Here's how the part is built. I have some questions about the finished solid (model axes, mm). A direction names the side the tool comes from. Round coordinates to 2 decimals unless told otherwise and drop trailing zeros. Loops run counter-clockwise (first coordinate to the right, second up) from the corner with the lowest first, then second, coordinate; pieces in that order, holes last. Notation, with made-up numbers: (75.5, -11) - (122.5, -11) arc R31 cw to (122.5, 25) - close; hole circle Ø1 at (-29.5, 56). An arc over 180 degrees is marked (long way). Answer as a JSON object with one key per item and string values. Group by question number.
1) Which directions (+Z, -Z, +X, -X, +Y, -Y) give clear straight access to the entire face, cutting with the end or side of a thin tool? Please do faces 1 (the face through (0, 15, 6)), 2 (the face through (0, 37, 12)), 3 (the face through (7, 45, 10)), 4 (the face through (10, 6.4, 5.9)).
2) I want a section at B-B, the plane y = 4. Please give me the cut outline in (x, z).
3) Will these pins go through, and if not, where does the flat tip stop? P1, Ø5, axis at x = 7, y = 28, coming from the +Z side; P2, Ø1.8, axis at x = 5.5, z = 8.5, coming from the +Y side; P3, Ø0.7, axis at x = -6, y = 44.5, coming from the +Z side; P4, Ø1.5, axis at x = -5.5, z = 3.5, coming from the +Y side.
4) I want a section at D-D, the plane y = 30. Please give me the cut outline in (x, z), then the cut area to 3 significant figures.
5) If I drill on line 1 along Y through (x, z) = (0, 3.5); line 2 along X through (y, z) = (44.5, 8.75); line 3 along X through (y, z) = (19, 10.5), over which ranges is the centre line in solid material (lowest first)? Write a range as [from, to].
6) If we mould it in two halves opening along Z, with no side actions, what happens to faces 5 (the face through (-12.535, 1.854, 6.676)), 6 (the face through (-6, 45, 7)), 7 (the face through (-10, 24, 6))? For each: pulls with the +Z half, pulls with the -Z half, needs draft (parallel to the pull), parting line crosses it, or undercut.
7) I want a section at A-A, the plane z = 6. Please give me the cut outline in (x, y), then the cut area to 3 significant figures.
8) I want a section at C-C, the plane x = 1.75. Please give me the cut outline in (y, z), then the cut area to 3 significant figures.
from build123d import *

# Parameters (mm, degrees)
SKETCH1_R           = 5
SKETCH1_W           = 20
SKETCH1_H           = 18
BOSS_EXTRUDE1_DEPTH = 12
SKETCH2_R           = 2.25
CUT_EXTRUDE1_DEPTH  = 69.14690015
SKETCH3_W           = 14
SKETCH3_H           = 3
CUT_EXTRUDE2_DEPTH  = 5


with BuildPart() as part:
    # Sketch1 → Boss-Extrude1 (new body)
    with BuildSketch(Plane.XY):
        with BuildLine():
            Line((15, 45), (15, 0))
            Line((15, 0), (10, 0))
            Line((10, 0), (10, 9))
            Line((10, 9), (-10, 9))
            Line((-10, 9), (-10, 0))
            Line((-10, 0), (-15, 0))
            Line((-15, 0), (-15, 45))
            ThreePointArc((-15, 45), (0, 60), (15, 45))
        make_face()
        with Locations((0, 45)):
            Circle(SKETCH1_R, mode=Mode.SUBTRACT)
        with Locations((0, 24)):
            Rectangle(SKETCH1_W, SKETCH1_H, mode=Mode.SUBTRACT)
    extrude(amount=BOSS_EXTRUDE1_DEPTH)

    # Sketch2 → Cut-Extrude1 (cut, through all)
    with BuildSketch(Plane.ZY.offset(15)):
        with Locations(Location((6, 4, 0), (0, 0, 270))):
            Circle(SKETCH2_R)
    extrude(amount=-CUT_EXTRUDE1_DEPTH, mode=Mode.SUBTRACT)

    # Sketch3 → Cut-Extrude2 (cut)
    with BuildSketch(Plane.XY.offset(12)):
        with Locations((0, 45)):
            Rectangle(SKETCH3_W, SKETCH3_H)
    extrude(amount=-CUT_EXTRUDE2_DEPTH, mode=Mode.SUBTRACT)


solid = part.part
Outcome:
{
 "1": {"face 1": "+Z, -Z", "face 2": "+Z, +X, -X, +Y, -Y", "face 3": "+Z", "face 4": "+Z, -Z, -Y"},
 "2": {"outline": "(-15, 0) - (-10, 0) - (-10, 3.75) - (-15, 3.75) - close; (-15, 8.25) - (-10, 8.25) - (-10, 12) - (-15, 12) - close; (10, 0) - (15, 0) - (15, 3.75) - (10, 3.75) - close; (10, 8.25) - (15, 8.25) - (15, 12) - (10, 12) - close"},
 "3": {"P1": "through", "P2": "y = 59.28", "P3": "z = 7", "P4": "y = 59.23"},
 "4": {"outline": "(-15, 0) - (-10, 0) - (-10, 12) - (-15, 12) - close; (10, 0) - (15, 0) - (15, 12) - (10, 12) - close", "area": "120 mm^2"},
 "5": {"line 1": "[9, 15], [33, 40], [50, 60]", "line 2": "[-15, -7], [7, 15]", "line 3": "[-15, -10], [10, 15]"},
 "6": {"face 5": "undercut", "face 6": "pulls with the +Z half", "face 7": "needs draft"},
 "7": {"outline": "(-15, 0) - (-10, 0) - (-10, 1.75) - (-15, 1.75) - close; (-15, 6.25) - (-10, 6.25) - (-10, 9) - (10, 9) - (10, 6.25) - (15, 6.25) - (15, 45) arc R15 ccw to (-15, 45) - close; (10, 0) - (15, 0) - (15, 1.75) - (10, 1.75) - close; hole (-10, 15) - (10, 15) - (10, 33) - (-10, 33) - close; hole circle Ø10 at (0, 45)", "area": "1,040 mm^2"},
 "8": {"outline": "(9, 0) - (15, 0) - (15, 12) - (9, 12) - close; (33, 0) - (40.32, 0) - (40.32, 12) - (33, 12) - close; (49.68, 0) - (59.9, 0) - (59.9, 12) - (49.68, 12) - close", "area": "282 mm^2"}
}
